Verification items for the finished model (mm, model axes). Face numbers are marked on the shaded views. A direction names the side the tool comes from. Coordinates: 2 decimals unless noted, no trailing zeros. Order: outer loops, then holes, each group sorted by start corner. A loop starts at its lowest first (then second) coordinate and runs counter-clockwise, first axis right, second up. Notation, with made-up numbers: (-17, -16) -> (6, -16) arc R13 ccw to (6, 8) -> close; hole circle Ø1 at (-4.75, 62.25). An arc over 180 degrees is marked (long way). Answer as CSV lines item,"result".
```python
from build123d import *

# Parameters (mm, degrees)
BOSS_EXTRUDE2_DEPTH = 1.5
FILLET1_R           = 2
BOSS_EXTRUDE3_DEPTH = 4.5
SKETCH1_3_R         = 0.63
SKETCH1_3_R_2       = 0.310429465
CUT_EXTRUDE2_DEPTH  = 15.345466183


with BuildPart() as part:
    # Sketch2 → Boss-Extrude2 (new, symmetric)
    with BuildSketch(Plane(origin=(0, 0, 0), x_dir=(0, 0, -1), z_dir=(1, 0, 0))):
        Polygon((-6, 12.5), (-6, 9.5), (-4.5, 9.5), (-2.22, 0), (0, 0), (-3, 12.5), align=None)
    boss_extrude2 = extrude(amount=BOSS_EXTRUDE2_DEPTH, both=True)

    # Fillet1
    fillet1_edges = [part.edges().sort_by_distance(p)[0] for p in [
        (0, 12.5, 3),
    ]]
    fillet(fillet1_edges, radius=FILLET1_R)

    # Sketch1 → Boss-Extrude3 (add)
    with BuildSketch(Plane(origin=(0, 0, 0), x_dir=(1, 0, 0), z_dir=(0, 1, 0))):
        with BuildLine():
            Line((-2.2, 1.48), (2.2, 1.48))
            ThreePointArc((2.2, 1.48), (3.68, 0), (2.2, -1.48))
            Line((2.2, -1.48), (-2.2, -1.48))
            ThreePointArc((-2.2, -1.48), (-3.68, 0), (-2.2, 1.48))
        make_face()
    extrude(amount=BOSS_EXTRUDE3_DEPTH)

    # Mirror1: Boss-Extrude2 across plane
    add(boss_extrude2.mirror(Plane.XY))

    # Sketch1_3 → Cut-Extrude2 (cut, through all)
    with BuildSketch(Plane(origin=(0, 0, 0), x_dir=(1, 0, 0), z_dir=(0, 1, 0))):
        with Locations(Location((-1.210810654, 0, 0), (0, 0, 270))):
            Circle(SKETCH1_3_R)
        with Locations(Location((1.453538454, 0.541981393, 0), (0, 0, 270))):
            Circle(SKETCH1_3_R_2)
        with Locations(Location((2.490372423, -0.541981393, 0), (0, 0, 270))):
            Circle(SKETCH1_3_R_2)
    extrude(amount=CUT_EXTRUDE2_DEPTH, mode=Mode.SUBTRACT)


solid = part.part
```
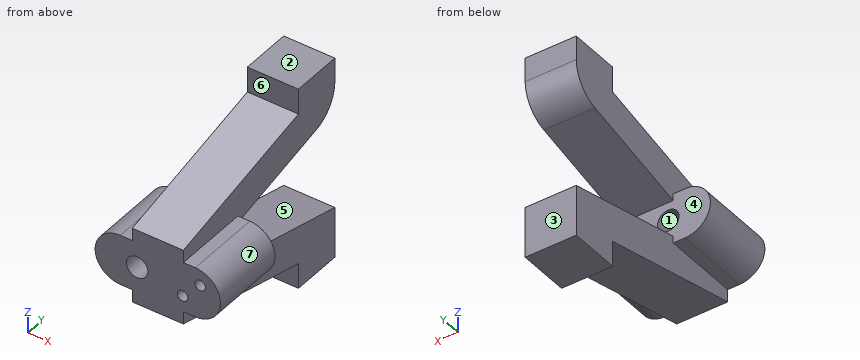
Item 1: Release check for a two-part mould opening along Z. For the marked faces 1, 2, 3 and 4 record: +Z half, -Z half, draft (parallel to the pull), parting line (faces both ways), or undercut.
Answer list:
face 1,"undercut"
face 2,"+Z half"
face 3,"draft"
face 4,"undercut"
Item 2: Section check A-A, the plane y = 5. Record the boundary of the cut face in (x, z).
Answer list:
outline,"(-1.5, -3.42) -> (1.5, -3.42) -> (1.5, -1.2) -> (-1.5, -1.2) -> close; (-1.5, 1.2) -> (1.5, 1.2) -> (1.5, 3.42) -> (-1.5, 3.42) -> close"
Item 3: Section check C-C, the plane x = -0.25. Record the boundary of the cut face in (y, z), plus the area to 3 significant figures.
Answer list:
outline,"(0, -2.22) -> (9.5, -4.5) -> (9.5, -6) -> (12.5, -6) -> (12.5, -3) -> (4.5, -1.08) -> (4.5, 1.08) -> (10.97, 2.63) arc R2 ccw to (12.5, 4.58) -> (12.5, 6) -> (9.5, 6) -> (9.5, 4.5) -> (0, 2.22) -> close"
area,"66.7 mm2"
Item 4: Section check D-D, the plane y = 3.25. Record the boundary of the cut face in (x, z), plus the area to 3 significant figures.
Answer list:
outline,"(-2.2, -1.48) -> (-1.5, -1.48) -> (-1.5, -3) -> (1.5, -3) -> (1.5, -1.48) -> (2.2, -1.48) arc R1.48 ccw to (2.2, 1.48) -> (1.5, 1.48) -> (1.5, 3) -> (-1.5, 3) -> (-1.5, 1.48) -> (-2.2, 1.48) arc R1.48 ccw to start; hole circle Ø1.26 at (-1.21, 0); hole circle Ø0.62 at (1.45, -0.54); hole circle Ø0.62 at (2.49, 0.54)"
area,"27.2 mm2"
Item 5: Depth check by flat-ended pin: pin 1 Ø3 at (x, y) = (1.5, 4.5) entering from +Z; pin 2 Ø2 at (x, y) = (-1, 4) entering from +Z; pin 3 Ø2.5 at (y, z) = (8.5, -3.5) entering from +X. Enter the tip coordinate at first touch or a pass-through.
Answer list:
pin 1,"z = 3.66"
pin 2,"z = 3.42"
pin 3,"x = 1.5"
Item 6: Thickness scan on line 1 (Y direction, x = -2.5, z = 0); line 2 (X direction, y = 2.65, z = 0); line 3 (Y direction, x = 1.25, z = -4.75). Record the ranges inside material, lowest first.
Answer list:
line 1,"0 to 4.5"
line 2,"-3.68 to -1.84, -0.58 to 3.68"
line 3,"9.5 to 12.5"
Item 7: Tool access check on the marked faces 5, 6 and 7. Record the directions out of +Z, -Z, +X, -X, +Y, -Y that give a thin tool (end or side, any length) a straight path to the whole face; none if there is none.
Answer list:
face 5,"+X, -X, +Y"
face 6,"+Z, +X, -X, -Y"
face 7,"+X, +Y, -Y"
Item 8: Section check B-B, the plane z = 0. Record the boundary of the cut face in (x, y), plus the area to 4 significant figures.
Answer list:
outline,"(-3.68, 0) -> (-1.84, 0) -> (-1.84, 4.5) -> (-3.68, 4.5) -> close; (-0.58, 0) -> (3.68, 0) -> (3.68, 4.5) -> (-0.58, 4.5) -> close"
area,"27.45 mm2"
